Autodesk Inventor part; units mm, degrees
ref_plane "YZ Plane" through (0, 0, 0) normal (1, 0, 0) x (0, 1, 0)
ref_plane "XZ Plane" through (0, 0, 0) normal (0, 1, 0) x (-1, 0, 0)
ref_plane "XY Plane" through (0, 0, 0) normal (0, 0, 1) x (1, 0, 0)
sketch "Sketch1" plane through (0, 0, 0) normal (1, 0, 0) x (0, 1, 0)
  line L0 (0, 0) -> (102.9, 0)
  line L1 (102.9, 0) -> (102.9, 10)
  line L2 (102.9, 10) -> (0, 10)
  line L3 (0, 10) -> (0, 0)
  line L4 (50, 10) -> (52.9, 10)
  line L5 (52.9, 10) -> (52.9, 5)
  line L6 (52.9, 5) -> (50, 5)
  line L7 (50, 5) -> (50, 10)
  line L8 (102.9, 10) -> (100, 10)
  line L9 (100, 10) -> (100, 5)
  line L10 (100, 5) -> (102.9, 5)
  line L11 (102.9, 5) -> (102.9, 10)
  line L12 (2.9, 5) -> (0, 5)
  line L13 (0, 5) -> (0, 10)
  line L14 (0, 10) -> (2.9, 10)
  line L15 (2.9, 10) -> (2.9, 5)
  line L16 (51.45, 5) -> (51.45, 0)
  point P0 (51.45, 10)
  dimension "d0" = 2.9
  dimension "d1" = 5
  dimension "d2" = 10
  dimension "d3" = 50
extrude "Extrusion1" add sketch "Sketch1" along normal blind 2.85 contours L3 L12 L15 L2 L7 L6 L16 L0 | L16 L6 L5 L2 L9 L10 L1 L0
fillet "Fillet1" radius 0.5 2 edges at (1.425, 0, 0) (1.425, 102.9, 0)
properties part number "comb_spacer"
Build history of the part. All positions in model axes, mm. A direction names the side the tool comes from. Round coordinates to 2 decimals unless told otherwise and drop trailing zeros. Write each loop counter-clockwise with the first axis right and the second up, starting at its lowest first coordinate (ties: lowest second). Pieces come first, ordered by that corner, then holes. Notation, with made-up numbers: M -1.75,81 L 39.25,81 A21 cw 39.25,88 Z; hole C 17.25,62.25 d1. An arc over 180 degrees is marked long. Answer in a Markdown table with one row per item.
1. Which spindle directions (+Z, -Z, +X, -X, +Y, -Y) get a long thin tool onto all of the face, cutting with end or side? Do faces 4 (the face through (1, 51, 0)), 5 (the face through (1, 101, 5)), 6 (the face through (2.85, 51, 4)), 7 (the face through (1, 1, 5)), 8 (the face through (1, 51, 5)). Say none if no direction does.
Geometry check:
| item | result |
|---|---|
| face 4 | -Z, +X, -X, +Y, -Y |
| face 5 | +Z, +X, -X, +Y |
| face 6 | +Z, -Z, +X, +Y, -Y |
| face 7 | +Z, +X, -X, -Y |
| face 8 | +Z, +X, -X |
2. Saw through at A-A (z = 6.25). List the corners of the cut face in (x, y).
Geometry check:
| item | result |
|---|---|
| outline | M 0,2.9 L 2.85,2.9 L 2.85,50 L 0,50 Z; M 0,52.9 L 2.85,52.9 L 2.85,100 L 0,100 Z |
3. Flat gauge pins, fed straight in: P1, Ø0.9, axis at x = 1, y = 101.5, coming from the +Z side; P2, Ø1.5, axis at x = 1.5, z = 5.5, coming from the -Y side; P3, Ø0.9, axis at x = 1, z = 6.5, coming from the -Y side. Where does each tip first touch, or does it go through?
Geometry check:
| item | result |
|---|---|
| P1 | z = 5 |
| P2 | y = 0 |
| P3 | y = 2.9 |
4. Mould opens along Y. For faces 1 (the face through (1, 102.9, 3)), 2 (the face through (1, 50, 7)), 3 (the face through (0, 51, 4)) say: +Y half, -Y half, draft (parallel to the pull), parting line (faces both ways), or undercut.
Geometry check:
| item | result |
|---|---|
| face 1 | +Y half |
| face 2 | undercut |
| face 3 | draft |
5. Saw through at B-B (x = 1.75). List the corners of the cut face in (y, z).
Geometry check:
| item | result |
|---|---|
| outline | M 0,0.5 A0.5 ccw 0.5,0 L 102.4,0 A0.5 ccw 102.9,0.5 L 102.9,5 L 100,5 L 100,10 L 52.9,10 L 52.9,5 L 50,5 L 50,10 L 2.9,10 L 2.9,5 L 0,5 Z |
6. Probe L1, parallel to Y at x = 2.6, z = 7.5. List the from-to ranges inside material, lowest first. Write a range as [from, to].
Geometry check:
| item | result |
|---|---|
| L1 | [2.9, 50], [52.9, 100] |
